```python
from build123d import *

# Parameters (mm, degrees)
F0_R     = 35
F1_DEPTH = 10
F2_R     = 22.5
F3_DEPTH = 5
F4_W     = 43
F4_H     = 14
F5_DEPTH = 5
F6_R     = 4
F7_DEPTH = 4.8


with BuildPart() as f1:
    # F0 (on Top) → F1 (new body)
    with BuildSketch(Plane.XY):
        Circle(F0_R)
    extrude(amount=F1_DEPTH)

    # F2 (on face) → F3 (cut)
    with BuildSketch(Plane(origin=(0, 0, 0), x_dir=(1, 0, 0), z_dir=(0, 0, -1))):
        Circle(F2_R)
    extrude(amount=-F3_DEPTH, mode=Mode.SUBTRACT)

    # F4 (on face) → F5 (cut)
    with BuildSketch(Plane.XY.offset(10)):
        with Locations((0, -17)):
            Rectangle(F4_W, F4_H)
    extrude(amount=-F5_DEPTH, mode=Mode.SUBTRACT)

    # F6 (on face) → F7 (cut)
    with BuildSketch(Plane.XY.offset(10)):
        Circle(F6_R)
    extrude(amount=-F7_DEPTH, mode=Mode.SUBTRACT)


solid = f1.part
```
Verification items for the finished model (mm, model axes). A direction names the side the tool comes from. Coordinates: 2 decimals unless noted, no trailing zeros. Order: outer loops, then holes, each group sorted by start corner. A loop starts at its lowest first (then second) coordinate and runs counter-clockwise, first axis right, second up. Notation, with made-up numbers: (81, 83.5) -> (119, 83.5) arc R16 ccw to (119, 89.5) -> close; hole circle Ø4 at (-22.75, 45.25). An arc over 180 degrees is marked (long way). Put each result on its own line as item: value. Start each with the question number.
1) Cross-section at D-D (x = 0). Enter the section's corners in (y, z), plus the area to 3 significant figures.
2) Cross-section at B-B (z = 9). Enter the section's corners in (x, y), plus the area to 3 significant figures.
3) Go/stop test with flat-tipped pins: pin 1 (1.5 mm diameter, centred on x = -8.5, z = 8, fed in from -Y); pin 2 (4 mm diameter, centred on y = -20.5, z = 7.5, fed in from -X); pin 3 (3 mm diameter, centred on y = 6, z = 3, fed in from +X); pin 4 (3 mm diameter, centred on x = 19.5, y = -26.5, fed in from -Z). Record where each tip stops, or that it passes through.
4) Release check for a two-part mould opening along Y. For faces 4 (the flat face through (0, -23, 5)), 5 (the flat face through (0, -23, 0)), 6 (the cylindrical face through (-28, -21, 5)), 7 (the flat face through (0, 0, 5.2)) record: pulls with the +Y half, pulls with the -Y half, needs draft (parallel to the pull), parting line crosses it, or undercut.
5) Material ranges on L1, parallel to Y at x = 0, z = 1.5; L2, parallel to Z at x = -7.5, y = 5.5; L3, parallel to Y at x = -19, z = 5.25, recorded low to high.
6) Cross-section at A-A (x = 11). Enter the section's corners in (y, z).
7) Cross-section at C-C (y = -5.5). Enter the section's corners in (x, z), plus the area to 3 significant figures.
8) Tool access check on faces 1 (the flat face through (0, 8, 10)), 2 (the cylindrical face through (-0.867, -3.905, 7.634)), 3 (the flat face through (0, 2, 5)). Record the directions out of +Z, -Z, +X, -X, +Y, -Y that give a thin tool (end or side, any length) a straight path to the whole face; none if there is none.
Geometry check:
1. outline: (-35, 0) -> (-22.5, 0) -> (-22.5, 5) -> (-24, 5) -> (-24, 10) -> (-35, 10) -> close; (-10, 5) -> (22.5, 5) -> (22.5, 0) -> (35, 0) -> (35, 10) -> (4, 10) -> (4, 5.2) -> (-4, 5.2) -> (-4, 10) -> (-10, 10) -> close
1. area: 367 mm^2
2. outline: circle Ø70 at (0, 0); hole (-21.5, -24) -> (21.5, -24) -> (21.5, -10) -> (-21.5, -10) -> close; hole circle Ø8 at (0, 0)
2. area: 3,200 mm^2
3. pin 1: stops at y = -34.13
3. pin 2: stops at x = -29.71
3. pin 3: stops at x = 34.71
3. pin 4: stops at z = 0
4. face 4: undercut
4. face 5: needs draft
4. face 6: parting line crosses it
4. face 7: undercut
5. L1: y = -35 to -22.5, 22.5 to 35
5. L2: z = 5 to 10
5. L3: y = -29.39 to -24, -10 to 29.39
6. outline: (-33.23, 0) -> (-19.63, 0) -> (-19.63, 5) -> (-24, 5) -> (-24, 10) -> (-33.23, 10) -> close; (-10, 5) -> (19.63, 5) -> (19.63, 0) -> (33.23, 0) -> (33.23, 10) -> (-10, 10) -> close
7. outline: (-34.57, 0) -> (-21.82, 0) -> (-21.82, 5) -> (21.82, 5) -> (21.82, 0) -> (34.57, 0) -> (34.57, 10) -> (-34.57, 10) -> close
7. area: 473 mm^2
8. face 1: +Z, +X, -X, +Y, -Y
8. face 2: +Z
8. face 3: -Z
